The listing builds one solid part. Answer for the finished solid, in the listing's coordinates (mm). A direction names the side the tool comes from. Coordinates: 2 decimals unless noted, no trailing zeros. Order: outer loops, then holes, each group sorted by start corner. A loop starts at its lowest first (then second) coordinate and runs counter-clockwise, first axis right, second up. Notation, with made-up numbers: (-31, 60) -> (14, 60) arc R17 ccw to (14, 69) -> close; hole circle Ø1 at (69.5, -35.75). An arc over 180 degrees is marked (long way). One line per question, with ' | ' between items.
from build123d import *

# Parameters (mm, degrees)
SKETCH1_W      = 9.8
SKETCH1_H      = 9.8
EXTRUDE1_DEPTH = 62
SKETCH2_R      = 1.5
EXTRUDE2_DEPTH = 10
EXTRUDE3_START = -10
SKETCH3_R      = 1.5
EXTRUDE3_DEPTH = 10
SKETCH4_R      = 1.55
EXTRUDE4_DEPTH = 10
SKETCH5_R      = 1.5
EXTRUDE5_DEPTH = 10
SKETCH6_W      = 9.8
SKETCH6_H      = 1
EXTRUDE6_DEPTH = 0.5


with BuildPart() as part:
    # Sketch1 → Extrude1 (new body)
    with BuildSketch(Plane(origin=(0, 0, 0), x_dir=(1, 0, 0), z_dir=(0, 1, 0))):
        Rectangle(SKETCH1_W, SKETCH1_H)
    extrude(amount=EXTRUDE1_DEPTH)

    # Sketch2 → Extrude2 (cut)
    with BuildSketch(Plane.XZ):
        with Locations(Location((0, 0, 0), (0, 0, 270))):
            Circle(SKETCH2_R)
    extrude(amount=-EXTRUDE2_DEPTH, mode=Mode.SUBTRACT)

    # Sketch3 → Extrude3 (cut)
    with BuildSketch(Plane(origin=(0, 62, 0), x_dir=(1, 0, 0), z_dir=(0, 1, 0)).offset(EXTRUDE3_START)):
        with Locations(Location((0, 0, 0), (0, 0, 90))):
            Circle(SKETCH3_R)
    extrude(amount=EXTRUDE3_DEPTH, mode=Mode.SUBTRACT)

    # Sketch4 → Extrude4 (cut)
    with BuildSketch(Plane(origin=(0, 0, -4.9), x_dir=(-1, 0, 0), z_dir=(0, 0, -1))):
        with Locations((0, 10)):
            Circle(SKETCH4_R)
        with Locations((0, 49)):
            Circle(SKETCH4_R)
        with Locations((0, 34)):
            Circle(SKETCH4_R)
        with Locations((0, 25)):
            Circle(SKETCH4_R)
    extrude(amount=-EXTRUDE4_DEPTH, mode=Mode.SUBTRACT)

    # Sketch5 → Extrude5 (cut)
    with BuildSketch(Plane.ZY.offset(4.9)):
        with Locations((0, 40)):
            Circle(SKETCH5_R)
        with Locations((0, 19)):
            Circle(SKETCH5_R)
    extrude(amount=-EXTRUDE5_DEPTH, mode=Mode.SUBTRACT)

    # Sketch6 → Extrude6 (cut)
    with BuildSketch(Plane.ZY.offset(4.9)):
        with Locations((0, 55.927600584)):
            Rectangle(SKETCH6_W, SKETCH6_H)
    extrude(amount=-EXTRUDE6_DEPTH, mode=Mode.SUBTRACT)


solid = part.part
Item 1: Section A-A, the plane y = 40 is taken. Give the vertices of the cut face in (x, z).
Computed values:
outline: (-4.9, -4.9) -> (4.9, -4.9) -> (4.9, -1.5) -> (-4.9, -1.5) -> close; (-4.9, 1.5) -> (4.9, 1.5) -> (4.9, 4.9) -> (-4.9, 4.9) -> close
Item 2: Find the intervals of material crossed by L1, parallel to Y at x = 0, z = 0; L2, parallel to Y at x = 0, z = 2; L3, parallel to Z at x = 0, y = 5.5, in increasing order.
Computed values:
L1: y = 11.55 to 17.5, 20.5 to 23.45, 26.55 to 32.45, 35.55 to 38.5, 41.5 to 47.45, 50.55 to 52 | L2: y = 0 to 8.45, 11.55 to 23.45, 26.55 to 32.45, 35.55 to 47.45, 50.55 to 62 | L3: z = -4.9 to -1.5, 1.5 to 4.9
Item 3: Section D-D, the plane z = -0.25 is taken. Give the vertices of the cut face in (x, y).
Computed values:
outline: (-4.9, 0) -> (-1.48, 0) -> (-1.48, 9.54) arc R1.55 cw (long way) to (1.48, 9.54) -> (1.48, 0) -> (4.9, 0) -> (4.9, 17.52) -> (-4.9, 17.52) -> close; (-4.9, 20.48) -> (4.9, 20.48) -> (4.9, 38.52) -> (-4.9, 38.52) -> close; (-4.9, 41.48) -> (4.9, 41.48) -> (4.9, 62) -> (1.48, 62) -> (1.48, 52) -> (-1.48, 52) -> (-1.48, 62) -> (-4.9, 62) -> (-4.9, 56.43) -> (-4.4, 56.43) -> (-4.4, 55.43) -> (-4.9, 55.43) -> close; hole circle Ø3.1 at (0, 25); hole circle Ø3.1 at (0, 34); hole circle Ø3.1 at (0, 49)
Item 4: This flat-tipped pin is pushed along its axis until it touches: pin 1 Ø2.5 at (x, z) = (0, 0) entering from +Y. Where does it stop, or does it pass through?
Computed values:
pin 1: stops at y = 52
Item 5: Section B-B, the plane x = 0 is taken. Count the separate pieces of the cut face and the enclosed holes in it, plus the area to 3 significant figures.
Computed values:
separate pieces: 6 | enclosed holes: 2 | area: 417 mm^2
Item 6: Section C-C, the plane z = 3.5 is taken. Give the vertices of the cut face in (x, y).
Computed values:
outline: (-4.9, 0) -> (4.9, 0) -> (4.9, 62) -> (-4.9, 62) -> (-4.9, 56.43) -> (-4.4, 56.43) -> (-4.4, 55.43) -> (-4.9, 55.43) -> close; hole circle Ø3.1 at (0, 10); hole circle Ø3.1 at (0, 25); hole circle Ø3.1 at (0, 34); hole circle Ø3.1 at (0, 49)
Item 7: For faces 1 (the face through (-0.45, 56.93, -1.43)), 2 (the face through (0.45, 4.74, -1.43)), 3 (the face through (-4.4, 56, 0)), 4 (the face through (0, 31, 4.9)), determine the directions among +Z, -Z, +X, -X, +Y, -Y from which every point of the face is accessible in a straight line to the end or side of a thin tool.
Computed values:
face 1: +Y | face 2: -Y | face 3: +Z, -Z, -X | face 4: +Z, +X, -X, +Y, -Y
Item 8: Determine the mould class of faces 5 (the face through (0, 31, -4.9)), 6 (the face through (-0.069, 38.536, -0.325)), 7 (the face through (4.9, 31, 0)), 8 (the face through (0, 52, 0)) for opening direction Z: pulls with the +Z half, pulls with the -Z half, needs draft (parallel to the pull), parting line crosses it, or undercut.
Computed values:
face 5: pulls with the -Z half | face 6: undercut | face 7: needs draft | face 8: undercut
